The model under review builds one solid part; all positions refer to its coordinate system, in mm. A direction names the side the tool comes from. Round coordinates to 2 decimals unless told otherwise and drop trailing zeros. Write each loop counter-clockwise with the first axis right and the second up, starting at its lowest first coordinate (ties: lowest second). Pieces come first, ordered by that corner, then holes. Notation, with made-up numbers: (39, 60) -> (75, 60) arc R13 ccw to (75, 73) -> close; hole circle Ø10 at (-19, 15.25). An arc over 180 degrees is marked (long way). Use CSV: the item, a comma, the result in double quotes. Start each with the question number.
1) For pin 1 Ø1.3 at (y, z) = (96.5, 3.5) entering from +X; pin 2 Ø1.8 at (x, y) = (-315, 94) entering from -Z; pin 3 Ø2 at (y, z) = (96.5, 4) entering from -X; pin 4 Ø3 at (x, z) = (-341.5, 2) entering from -Y, all flat-tipped, find the tip position at first contact; note any pin that passes through.
2) Wall thickness on probe 1 along Y at (x, z) = (-312, 4.4); probe 2 along Y at (x, z) = (-328, 4.1); probe 3 along X at (y, z) = (56.5, 2.1): over which ranges is each line inside the solid? List them lowest first. Write a range as [from, to].
3) Take a section at A-A, the plane x = -312. Give the boundary of the cut face in (y, z).
4) Take a section at D-D, the plane x = -369. Give the boundary of the cut face in (y, z), then the cut area to 3 significant figures.
5) Mouldability with a two-part tool opening along X and no side actions: class faces 4 (the face through (-302.85, 23.01, 2.96)), 5 (the face through (-391.99, 22.85, 2.96)), 6 (the face through (-316.246, 60.187, 2.958)), 7 (the face through (-347, 61, 6)) as released by +X, released by -X, zero draft, split by the parting line, or undercut.
6) Machinability: for faces 1 (the face through (-315, 22, 3)), 2 (the face through (-380, 98, 3)), 3 (the face through (-313.905, 27.025, 3.042)), which of the approach directions +Z, -Z, +X, -X, +Y, -Y give a long, thin tool a straight path to every point of the face, cutting with its end or side? Answer none if there is none.
7) Take a section at B-B, the plane y = 60. Give the boundary of the cut face in (x, z).
8) Take a section at C-C, the plane z = 5. Give the boundary of the cut face in (x, y).
from build123d import *

# Parameters (mm, degrees)
SKETCH1_R           = 4.25
BOSS_EXTRUDE1_DEPTH = 6
SKETCH2_R           = 1.5
CUT_EXTRUDE1_DEPTH  = 7


with BuildPart() as part:
    # Sketch1 → Boss-Extrude1 (new body)
    with BuildSketch(Plane.XY):
        with BuildLine():
            Line((-380, 94), (-315, 94))
            Line((-315, 94), (-315, 100))
            Line((-315, 100), (-310, 100))
            ThreePointArc((-310, 100), (-302.928932188, 97.071067812), (-300, 90))
            Line((-300, 90), (-300, 30))
            ThreePointArc((-300, 30), (-302.928932188, 22.928932188), (-310, 20))
            Line((-310, 20), (-315, 20))
            Line((-315, 20), (-315, 26))
            Line((-315, 26), (-380, 26))
            Line((-380, 26), (-380, 20))
            Line((-380, 20), (-385, 20))
            ThreePointArc((-385, 20), (-392.071067812, 22.928932188), (-395, 30))
            Line((-395, 30), (-395, 90))
            ThreePointArc((-395, 90), (-392.071067812, 97.071067812), (-385, 100))
            Line((-385, 100), (-380, 100))
            Line((-380, 100), (-380, 94))
        make_face()
        with Locations((-312, 60)):
            Circle(SKETCH1_R, mode=Mode.SUBTRACT)
        with Locations((-383, 60)):
            Circle(SKETCH1_R, mode=Mode.SUBTRACT)
    extrude(amount=BOSS_EXTRUDE1_DEPTH)

    # Sketch2 → Cut-Extrude1 (cut, through all)
    with BuildSketch(Plane.XY.offset(6)):
        with Locations((-380, 26)):
            Circle(SKETCH2_R)
        with Locations((-315, 26)):
            Circle(SKETCH2_R)
        with Locations((-380, 94)):
            Circle(SKETCH2_R)
        with Locations((-315, 94)):
            Circle(SKETCH2_R)
    extrude(amount=-CUT_EXTRUDE1_DEPTH, mode=Mode.SUBTRACT)


solid = part.part
Values found:
1,pin 1,"x = -301.89"
1,pin 2,"through"
1,pin 3,"x = -393.35"
1,pin 4,"y = 26"
2,probe 1,"[20, 55.75], [64.25, 100]"
2,probe 2,"[26, 94]"
2,probe 3,"[-395, -385.41], [-380.59, -314.41], [-309.59, -300]"
3,outline,"(20, 0) -> (55.75, 0) -> (55.75, 6) -> (20, 6) -> close; (64.25, 0) -> (100, 0) -> (100, 6) -> (64.25, 6) -> close"
4,outline,"(26, 0) -> (94, 0) -> (94, 6) -> (26, 6) -> close"
4,area,"408 mm²"
5,face 4,"released by +X"
5,face 5,"released by -X"
5,face 6,"undercut"
5,face 7,"zero draft"
6,face 1,"+Z, -Z, -Y"
6,face 2,"+Z, -Z, +Y"
6,face 3,"+Z, -Z"
7,outline,"(-395, 0) -> (-387.25, 0) -> (-387.25, 6) -> (-395, 6) -> close; (-378.75, 0) -> (-316.25, 0) -> (-316.25, 6) -> (-378.75, 6) -> close; (-307.75, 0) -> (-300, 0) -> (-300, 6) -> (-307.75, 6) -> close"
8,outline,"(-395, 30) arc R10 ccw to (-385, 20) -> (-380, 20) -> (-380, 24.5) arc R1.5 cw (long way) to (-378.5, 26) -> (-316.5, 26) arc R1.5 cw (long way) to (-315, 24.5) -> (-315, 20) -> (-310, 20) arc R10 ccw to (-300, 30) -> (-300, 90) arc R10 ccw to (-310, 100) -> (-315, 100) -> (-315, 95.5) arc R1.5 cw (long way) to (-316.5, 94) -> (-378.5, 94) arc R1.5 cw (long way) to (-380, 95.5) -> (-380, 100) -> (-385, 100) arc R10 ccw to (-395, 90) -> close; hole circle Ø8.5 at (-383, 60); hole circle Ø8.5 at (-312, 60)"
